Work out the finished part from the listing and answer in its coordinate system (mm). A direction names the side the tool comes from. Round coordinates to 2 decimals unless told otherwise and drop trailing zeros. Loops run counter-clockwise (first coordinate to the right, second up) from the corner with the lowest first, then second, coordinate; pieces in that order, holes last. Notation, with made-up numbers: (-25, -9.75) - (32, -9.75) arc R13 cw to (32, 12.25) - close; hole circle Ø11 at (21, 12). An arc over 180 degrees is marked (long way). Answer as CSV lines item,"result". Start each with the question number.
Autodesk Inventor part; units mm, degrees
ref_plane "YZ Plane" through (0, 0, 0) normal (1, 0, 0) x (0, 1, 0)
ref_plane "XZ Plane" through (0, 0, 0) normal (0, 1, 0) x (-1, 0, 0)
ref_plane "XY Plane" through (0, 0, 0) normal (0, 0, 1) x (1, 0, 0)
sketch "Sketch1" plane through (0, 0, 0) normal (0, 0, 1) x (1, 0, 0)
  line L0 (0, 20) -> (0, -20)
  line L1 (0, 20) -> (-20, 20)
  arc A0 (-20, 20) -> (-20, -20) centre (-20, 0) ccw
  line L2 (-20, -20) -> (0, -20)
  point P0 (0, 0)
  point P1 (0, 0)
  dimension "d0" = 20
  dimension "d1" = 20
extrude "Extrusion1" add sketch "Sketch1" along normal blind 6
sketch "Sketch2" plane through (0, 0, 6) normal (0, 0, 1) x (1, 0, 0)
  circle A0 centre (-20, 0) radius 17.5 construction
  line L0 (0, -20) -> (0, 20)
  point P0 (0, 0)
  point P1 (0, 0)
  point P2 (-37.5, 0)
  point P3 (0, 0)
  dimension "d5" = 35
  dimension "d4" = 20
hole "Hole1" at (-37.5, 0, 6) direction (0, 0, -1) diameter 2.459 depth 6
pattern_circular "Circular Pattern1" count 5 over 360 about axis through (-20, 0, 0) along (0, 0, 1) of "Hole1"
sketch "Sketch4" plane through (0, -20, 0) normal (1, 0, 0) x (0, 0, -1)
  line L0 (0, 0) -> (0, 40)
  line L1 (0, 40) -> (-6, 40)
  point P0 (0, 20)
  point P1 (-3, 36)
  point P2 (-3, 20)
  point P3 (-3, 4)
  point P4 (0, 20)
  point P5 (-3, 40)
  dimension "d16" = 32
  dimension "d17" = 16
hole "Hole2" at (0, 16, 3) at (0, -16, 3) direction (-1, 0, 0) diameter 4.134 depth 14.2
hole "Hole3" at (0, 0, 3) direction (-1, 0, 0) diameter 4.134 depth 14.2
sketch "Sketch5" plane through (0, 0, 6) normal (0, 0, 1) x (1, 0, 0)
  circle A0 centre (-20, 0) radius 15
  line L0 (0, -20) -> (0, 20)
  arc A1 (-20, 20) -> (-20, -20) centre (-20, 0) ccw
  point P0 (0, 0)
  point P1 (0, 0)
  point P2 (0, 0)
  dimension "d32" = 30
extrude "Extrusion2" cut sketch "Sketch5" against normal up to surface (6 mm away)
properties part number "34" material "Gold"
Item 1: Section B-B, the plane x = -8.5 is taken. Give the vertices of the cut face in (y, z).
Item 2: Section C-C, the plane y = -16 is taken. Give the vertices of the cut face in (x, z).
Item 3: Find the intervals of material crossed by L1, parallel to Y at x = -3.8, z = 3; L2, parallel to Z at x = -8, y = 16; L3, parallel to Y at x = -26, z = 2, in increasing order.
Item 4: Which of the six approach directions +Z, -Z, +X, -X, +Y, -Y give full straight-line access (tool end or side, diameter ignored) to faces 1 (the face through (-7, 9, 6)), 2 (the face through (-7.2, -18.05, 3.27))?
Item 5: Determine the mould class of faces 3 (the face through (-7, 9, 0)), 4 (the face through (-5.39, 11.43, 2.96)), 5 (the face through (-10, -20, 3)) for opening direction Y: pulls with the +Y half, pulls with the -Y half, needs draft (parallel to the pull), parting line crosses it, or undercut.
Item 6: Flat-ended cylindrical pins translate along their axes: pin 1 Ø3.5 at (y, z) = (0, 3) entering from -X; pin 2 Ø3.5 at (y, z) = (16, 3) entering from +X; pin 3 Ø1 at (y, z) = (5.5, 1.5) entering from -X. Find the tip coordinate at first contact, or state that the pin passes through.
Item 7: Section D-D, the plane x = -20.5 is taken. Give the vertices of the cut face in (y, z).
Item 8: Section A-A, the plane y = 0 is taken. Give the vertices of the cut face in (x, z).
Answer:
1,outline,"(-20, 0) - (-9.63, 0) - (-9.63, 6) - (-20, 6) - close; (9.63, 0) - (20, 0) - (20, 6) - (9.63, 6) - close; hole circle Ø4.13 at (-16, 3); hole circle Ø4.13 at (16, 3)"
2,outline,"(-32, 0) - (-26.46, 0) - (-26.46, 6) - (-32, 6) - close; (-24.36, 0) - (0, 0) - (0, 0.93) - (-14.2, 0.93) - (-14.2, 5.07) - (0, 5.07) - (0, 6) - (-24.36, 6) - close"
3,L1,"y = -20 to -18.07, -13.93 to -2.07, 2.07 to 13.93, 18.07 to 20"
3,L2,"z = 0 to 0.93, 5.07 to 6"
3,L3,"y = -19.08 to -17.72, -15.57 to -13.75, 13.75 to 15.57, 17.72 to 19.08"
4,face 1,"+Z, +X, -X, +Y, -Y"
4,face 2,"+X"
5,face 3,"needs draft"
5,face 4,"undercut"
5,face 5,"pulls with the -Y half"
6,pin 1,"stops at x = -40"
6,pin 2,"stops at x = -14.2"
6,pin 3,"stops at x = -39.36"
7,outline,"(-19.99, 0) - (-14.99, 0) - (-14.99, 6) - (-19.99, 6) - close; (14.99, 0) - (19.99, 0) - (19.99, 6) - (14.99, 6) - close"
8,outline,"(-40, 0) - (-38.73, 0) - (-38.73, 6) - (-40, 6) - close; (-36.27, 0) - (-35, 0) - (-35, 6) - (-36.27, 6) - close; (-5, 0) - (0, 0) - (0, 0.93) - (-5, 0.93) - close; (-5, 5.07) - (0, 5.07) - (0, 6) - (-5, 6) - close"
